Print and shaded views of the part. All mm, measured from the part's lowest x, y and z. A direction names the side the tool comes from. Give positions to 0.01 mm unless a question says otherwise; leave off trailing zeros. Loops run counter-clockwise (first coordinate to the right, second up) from the corner with the lowest first, then second, coordinate; pieces in that order, holes last. Notation, with made-up numbers: M -5.75,37.5 L 31.25,37.5 A5 cw 31.25,43.5 Z; hole C -27,14.25 d10. An arc over 180 degrees is marked long. Put each result on its own line as item: value. Start each with the question number.
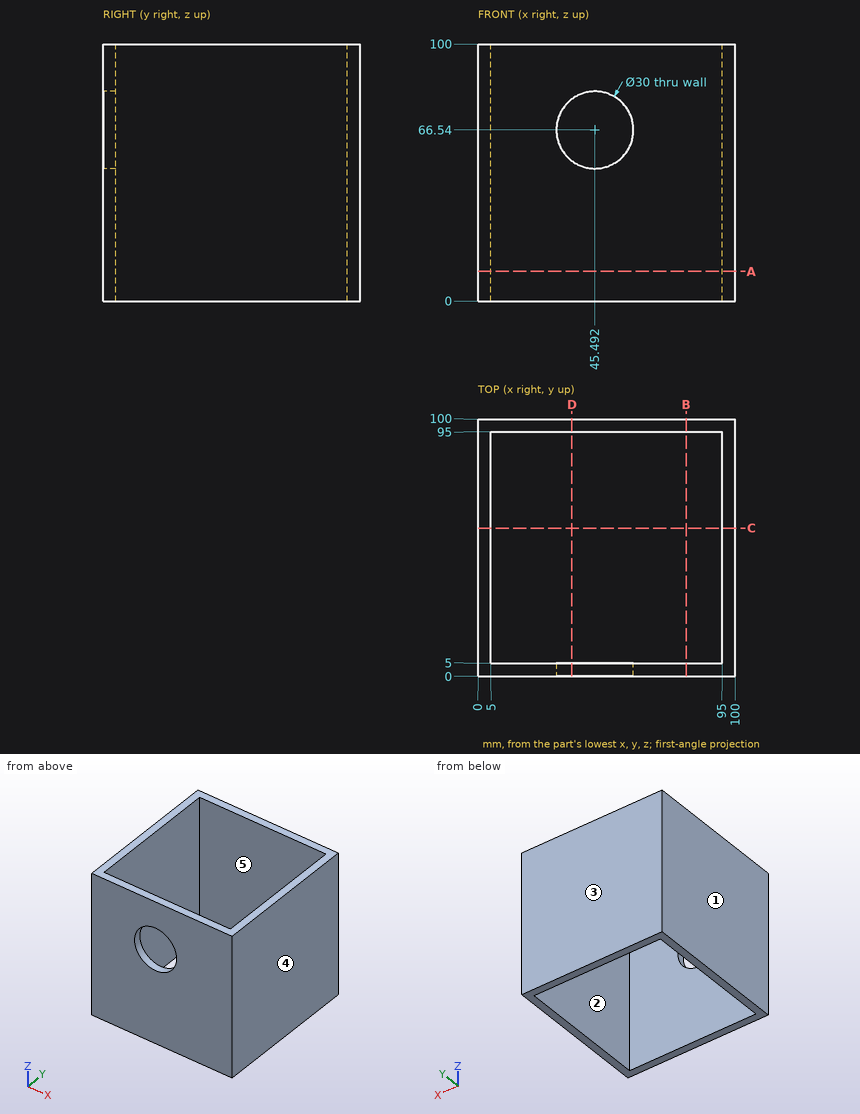
1) Band-saw the part on D-D on x = 36.5. Give the cut face in (y, z).
2) Band-saw the part on B-B on x = 81. Give the cut face in (y, z), then the cut area to 3 significant figures.
3) Pin check, flat tips, straight feed: pin 1 Ø1 at (y, z) = (75, 42.5) entering from -X; pin 2 Ø6 at (x, z) = (53, 59) entering from -Y. Stop position of each tip, or through.
4) Band-saw the part on A-A on z = 11.5. Give the cut face in (x, y).
5) Mould opens along Y. For the marked faces 1, 2 and 3 say: +Y half, -Y half, draft (parallel to the pull), parting line (faces both ways), or undercut.
6) Wall check: L1, parallel to Y at x = 13.5, z = 85.5; L2, parallel to X at y = 4, z = 69 (1 decimal). Give the ranges that are in metal, low to high.
7) Which spindle directions (+Z, -Z, +X, -X, +Y, -Y) get a long thin tool onto all of the face, cutting with end or side? Do the marked faces 4 and 5. Say none if no direction does.
Evaluation:
1. outline: M 0,0 L 5,0 L 5,54.53 L 0,54.53 Z; M 0,78.55 L 5,78.55 L 5,100 L 0,100 Z; M 95,0 L 100,0 L 100,100 L 95,100 Z
2. outline: M 0,0 L 5,0 L 5,100 L 0,100 Z; M 95,0 L 100,0 L 100,100 L 95,100 Z
2. area: 1,000 mm2
3. pin 1: x = 0
3. pin 2: y = 95
4. outline: M 0,0 L 100,0 L 100,100 L 0,100 Z; hole M 5,5 L 95,5 L 95,95 L 5,95 Z
5. face 1: draft
5. face 2: undercut
5. face 3: +Y half
6. L1: 0 to 5, 95 to 100
6. L2: 0 to 30.7, 60.3 to 100
7. face 4: +Z, -Z, +X, +Y, -Y
7. face 5: +Z, -Z
